The model under review builds one solid part; all positions refer to its coordinate system, in mm. A direction names the side the tool comes from. Give positions to 0.01 mm unless a question says otherwise; leave off trailing zeros. Loops run counter-clockwise (first coordinate to the right, second up) from the corner with the lowest first, then second, coordinate; pieces in that order, holes last. Notation, with made-up numbers: (54.25, -11) - (80.25, -11) arc R24 cw to (80.25, 25) - close; hole circle Ø6 at (78, 28.5). An arc over 180 degrees is marked (long way). Answer as a JSON object with one key per item and string values.
from build123d import *

# Parameters (mm, degrees)
F0_W     = 24.5
F0_H     = 24.5
F0_R     = 9.25
F1_DEPTH = 14
F2_R     = 2.2
F3_DEPTH = 24.5
F2_R_2   = 4.1
F4_DEPTH = 24.5
F5_START = -3
F5_DEPTH = 21.5
F6_SIZE  = 5


# Not quite as in the source:
# - a feature of the source that left no trace in its solid (it failed there, or was rolled back) is left out


with BuildPart() as f1:
    # F0 (on Top) → F1 (new body)
    with BuildSketch(Plane.XY):
        Rectangle(F0_W, F0_H)
        Circle(F0_R, mode=Mode.SUBTRACT)
    extrude(amount=F1_DEPTH)

    # F2 (on face) → F3 (cut, through all)
    with BuildSketch(Plane(origin=(0, 12.25, 0), x_dir=(-1, 0, 0), z_dir=(0, 1, 0))):
        with Locations((0, 7)):
            Circle(F2_R)
    extrude(amount=-F3_DEPTH, mode=Mode.SUBTRACT)

    # F2 (on face) → F4 (join, through all)
    with BuildSketch(Plane(origin=(0, 12.25, 0), x_dir=(-1, 0, 0), z_dir=(0, 1, 0))):
        with BuildLine():
            Line((-12.25, 7), (-12.25, 14))
            Line((-12.25, 14), (-16.35, 14))
            ThreePointArc((-16.35, 14), (-23.35, 7), (-16.35, 0))
            Line((-16.35, 0), (-12.25, 0))
            Line((-12.25, 0), (-12.25, 7))
        make_face()
        with Locations((-16.35, 7)):
            Circle(F2_R_2, mode=Mode.SUBTRACT)
        with Locations((-16.35, 7)):
            Circle(F2_R_2)
    extrude(amount=-F4_DEPTH)

    # F2 (on face) → F5 (cut)
    with BuildSketch(Plane(origin=(0, 12.25, 0), x_dir=(-1, 0, 0), z_dir=(0, 1, 0)).offset(F5_START)):
        with Locations((-16.35, 7)):
            Circle(F2_R_2)
    extrude(amount=-F5_DEPTH, mode=Mode.SUBTRACT)

    # F6
    f6_edges = [f1.edges().sort_by_distance(p)[0] for p in [
        (-12.25, 12.25, 7),
        (-12.25, -12.25, 7),
    ]]
    chamfer(f6_edges, length=F6_SIZE)


solid = f1.part
Q1. Clearance check with flat-ended pins moving along their axes: pin 1 Ø12 at (x, y) = (0.5, -8.5) entering from -Z; pin 2 Ø6 at (y, z) = (-0.5, 3) entering from +X; pin 3 Ø2.5 at (x, z) = (15.5, 6.5) entering from -Y. State where each tip first meets the part, or that it passes through.
Results:
{"pin 1": "stops at z = 0", "pin 2": "stops at x = 23.28", "pin 3": "stops at y = 9.25"}
Q2. Consider section A-A, the plane y = -3. State the section outline as (x, z) points.
Results:
{"outline": "(-12.25, 0) - (-8.75, 0) - (-8.75, 14) - (-12.25, 14) - close; (8.75, 0) - (16.35, 0) arc R7 ccw to (16.35, 14) - (8.75, 14) - close; hole circle Ø8.2 at (16.35, 7)"}
Q3. Consider section D-D, the plane x = 6. State the section outline as (y, z) points.
Results:
{"outline": "(-12.25, 0) - (-7.04, 0) - (-7.04, 14) - (-12.25, 14) - close; (7.04, 0) - (12.25, 0) - (12.25, 14) - (7.04, 14) - close"}
Q4. For faces 5 (the face through (-9.8, 9.7, 6.9)), 6 (the face through (12.563, -1.349, 5.43)), list the 3-axis set-ups (+Z, -Z, +X, -X, +Y, -Y) from which the entire face can be reached by the end or side of a thin tool; tool diameter is ignored.
Results:
{"face 5": "+Z, -Z, -X, +Y", "face 6": "-Y"}
Q5. To check wall thickness, follow probe 1 along Z at (x, y) = (0, 10.6); probe 2 along X at (y, z) = (2, 7.75); probe 3 along X at (y, z) = (7.25, 1). State the ranges of each line that lie inside material, in increasing order. Write a range as [from, to].
Results:
{"probe 1": "z = [0, 4.8], [9.2, 14]", "probe 2": "x = [-12.25, -9.03], [9.03, 12.32], [20.38, 23.31]", "probe 3": "x = [-12.25, -5.74], [5.74, 19.96]"}
Q6. The part is to be moulded in two halves that separate along Y. For faces 1 (the face through (9, 6, 0)), 2 (the face through (4.268, -8.206, 6.902)), 3 (the face through (-9.7, -9.8, 6.9)), 4 (the face through (8, 12.25, 7)), say which applies: +Y half, -Y half, draft (parallel to the pull), parting line (faces both ways), or undercut.
Results:
{"face 1": "draft", "face 2": "undercut", "face 3": "-Y half", "face 4": "+Y half"}
Q7. Consider section B-B, the plane x = 0. State the section outline as (y, z) points.
Results:
{"outline": "(-12.25, 0) - (-9.25, 0) - (-9.25, 4.8) - (-12.25, 4.8) - close; (-12.25, 9.2) - (-9.25, 9.2) - (-9.25, 14) - (-12.25, 14) - close; (9.25, 0) - (12.25, 0) - (12.25, 4.8) - (9.25, 4.8) - close; (9.25, 9.2) - (12.25, 9.2) - (12.25, 14) - (9.25, 14) - close"}
Q8. Consider section C-C, the plane z = 7. State the section outline as (x, y) points, plus the area to 3 significant figures.
Results:
{"outline": "(-12.25, -7.25) - (-7.25, -12.25) - (-2.2, -12.25) - (-2.2, -8.98) arc R9.25 cw to (-2.2, 8.98) - (-2.2, 12.25) - (-7.25, 12.25) - (-12.25, 7.25) - close; (2.2, -12.25) - (12.25, -12.25) - (12.25, 9.25) - (20.45, 9.25) - (20.45, -12.25) - (23.35, -12.25) - (23.35, 12.25) - (2.2, 12.25) - (2.2, 8.98) arc R9.25 cw to (2.2, -8.98) - close", "area": "375 mm^2"}
